Source: CAD feature listing. Evaluate the final solid. Frame: model axes, mm. A direction names the side the tool comes from. Give positions to 0.01 mm unless a question says otherwise; leave off trailing zeros. Loops run counter-clockwise (first coordinate to the right, second up) from the corner with the lowest first, then second, coordinate; pieces in that order, holes last. Notation, with made-up numbers: M -36,84.25 L -16,84.25 A24 ccw -16,114.25 Z; hole C -0.75,25 d3. An arc over 180 degrees is marked long. Answer in a Markdown table with one row per item.
```python
from build123d import *

# Parameters (mm, degrees)
F0_R     = 1.45
F0_R_2   = 2.24
F0_R_3   = 4.865
F0_R_4   = 3.415
F1_DEPTH = 18.64
F3_DEPTH = 9.2
F4_R     = 2.24
F5_DEPTH = 2
F6_W     = 4.65
F6_H     = 5.0977936404
F7_DEPTH = 8.93


with BuildPart() as f1:
    # F0 (on Top) → F1 (new body)
    with BuildSketch(Plane.XY):
        with BuildLine():
            Line((-53.71, -11.11), (5.8, -11.11))
            ThreePointArc((5.8, -11.11), (9.3355339059, -9.6455339059), (10.8, -6.11))
            Line((10.8, -6.11), (10.8, 6.11))
            ThreePointArc((10.8, 6.11), (9.3355339059, 9.6455339059), (5.8, 11.11))
            Line((5.8, 11.11), (-53.71, 11.11))
            Line((-53.71, 11.11), (-53.71, -11.11))
        make_face()
        with Locations((-20.01, -8.72)):
            Circle(F0_R, mode=Mode.SUBTRACT)
        with Locations((-11.43, 0)):
            Circle(F0_R_2, mode=Mode.SUBTRACT)
        Circle(F0_R_3, mode=Mode.SUBTRACT)
        with Locations((-20.01, 8.72)):
            Circle(F0_R, mode=Mode.SUBTRACT)
        Circle(F0_R_3)
        Circle(F0_R_4, mode=Mode.SUBTRACT)
        Circle(F0_R_4)
        with Locations((-11.43, 0)):
            Circle(F0_R_2)
    extrude(amount=F1_DEPTH)

    # F2 (on face) → F3 (join)
    with BuildSketch(Plane.XY.offset(18.64)):
        with BuildLine():
            Line((-2.325, 2.5488968202), (-2.325, -2.5488968202))
            ThreePointArc((-2.325, -2.5488968202), (0, -3.45), (2.325, -2.5488968202))
            Line((2.325, -2.5488968202), (2.325, 2.5488968202))
            Line((2.325, 2.5488968202), (-2.325, 2.5488968202))
        make_face()
        with BuildLine():
            ThreePointArc((2.325, 2.5488968202), (0, 3.45), (-2.325, 2.5488968202))
            Line((-2.325, 2.5488968202), (2.325, 2.5488968202))
        make_face()
    extrude(amount=F3_DEPTH)

    # F4 (on face) → F5 (join)
    with BuildSketch(Plane.XY.offset(18.64)):
        with Locations((-11.43, 0)):
            Circle(F4_R)
    extrude(amount=F5_DEPTH)

    # F6 (on face) → F7 (join)
    with BuildSketch(Plane.XY):
        with BuildLine():
            Line((-2.325, 2.5488968202), (2.325, 2.5488968202))
            ThreePointArc((2.325, 2.5488968202), (0, 3.45), (-2.325, 2.5488968202))
        make_face()
        with BuildLine():
            ThreePointArc((-2.325, -2.5488968202), (0, -3.45), (2.325, -2.5488968202))
            Line((2.325, -2.5488968202), (-2.325, -2.5488968202))
        make_face()
        Rectangle(F6_W, F6_H)
    extrude(amount=-F7_DEPTH)


solid = f1.part
```
Q1. Section query B-B (x = -20.01). Output: boundary loops of the cut face in (y, z).
Values follow:
| item | result |
|---|---|
| outline | M -11.11,0 L -10.17,0 L -10.17,18.64 L -11.11,18.64 Z; M -7.27,0 L 7.27,0 L 7.27,18.64 L -7.27,18.64 Z; M 10.17,0 L 11.11,0 L 11.11,18.64 L 10.17,18.64 Z |
Q2. Mould query, pull axis Y, two halves, no side actions, for faces 1 (the cylindrical face through (-21.08, 9.7, 9.19)), 2 (the cylindrical face through (-21.46, -8.66, 9.19)), 3 (the flat face through (-22, 0, 18.64)), 4 (the cylindrical face through (9.3, -9.68, 9.19)). Classes: +Y half, -Y half, draft (parallel to the pull), parting line (faces both ways), or undercut.
Values follow:
| item | result |
|---|---|
| face 1 | undercut |
| face 2 | undercut |
| face 3 | draft |
| face 4 | -Y half |
Q3. Section query C-C (y = 0). Output: boundary loops of the cut face in (x, z) (3 decimals).
Values follow:
| item | result |
|---|---|
| outline | M -53.71,0 L -2.325,0 L -2.325,-8.93 L 2.325,-8.93 L 2.325,0 L 10.8,0 L 10.8,18.64 L 2.325,18.64 L 2.325,27.84 L -2.325,27.84 L -2.325,18.64 L -9.19,18.64 L -9.19,20.64 L -13.67,20.64 L -13.67,18.64 L -53.71,18.64 Z |
Q4. Reachability of faces 5 (the flat face through (2.325, 0, -4)), 6 (the flat face through (-11, 0, 20.64)), 7 (the cylindrical face through (-0.04, -3.45, -4.4)) from +Z, -Z, +X, -X, +Y, -Y: full face, straight path, thin tool, end or side. Return the list, or none.
Values follow:
| item | result |
|---|---|
| face 5 | -Z, +X, +Y, -Y |
| face 6 | +Z, -X, +Y, -Y |
| face 7 | -Z, -Y |
Q5. Contact query for flat-ended pins moving along their axis: pin 1 Ø4 at (y, z) = (-0.5, 25) entering from -X (3 decimals); pin 2 Ø3.5 at (x, y) = (-11, 0.5) entering from +Z; pin 3 Ø6.5 at (x, y) = (-23.5, 1) entering from +Z; pin 4 Ø10 at (y, z) = (-8, 20.5) entering from -X. Output: stop coordinate, or through.
Values follow:
| item | result |
|---|---|
| pin 1 | x = -2.325 |
| pin 2 | z = 20.64 |
| pin 3 | z = 18.64 |
| pin 4 | x = -53.71 |
Q6. Ray query, probe 1 along Y at (x, z) = (-20.01, 13); probe 2 along X at (y, z) = (-6.5, 4); probe 3 along Z at (x, y) = (-18, 1.5). Return the intervals inside material, ascending. Write a range as from..to.
Values follow:
| item | result |
|---|---|
| probe 1 | -11.11..-10.17, -7.27..7.27, 10.17..11.11 |
| probe 2 | -53.71..10.78 |
| probe 3 | 0..18.64 |
Q7. Section query A-A (z = 8). Output: boundary loops of the cut face in (x, y).
Values follow:
| item | result |
|---|---|
| outline | M -53.71,-11.11 L 5.8,-11.11 A5 ccw 10.8,-6.11 L 10.8,6.11 A5 ccw 5.8,11.11 L -53.71,11.11 Z; hole C -20.01,-8.72 d2.9; hole C -20.01,8.72 d2.9 |
Q8. Section query D-D (y = 8.72). Output: boundary loops of the cut face in (x, z), plus the area to 3 significant figures.
Values follow:
| item | result |
|---|---|
| outline | M -53.71,0 L -21.46,0 L -21.46,18.64 L -53.71,18.64 Z; M -18.56,0 L 10.06,0 L 10.06,18.64 L -18.56,18.64 Z |
| area | 1,130 mm^2 |
